```python
from build123d import *

# Parameters (mm, degrees)
SKETCH1_R           = 4
BOSS_EXTRUDE1_DEPTH = 3.175
SKETCH2_R           = 12.7
SKETCH2_R_2         = 10.287
EXTRUDE_THIN1_DEPTH = 38.1
SKETCH3_R           = 12.7
SKETCH3_R_2         = 12.5
CUT_EXTRUDE2_DEPTH  = 19.05
SKETCH4_R           = 12.5
SKETCH4_R_2         = 11.95
CUT_EXTRUDE3_DEPTH  = 1.55


with BuildPart() as part:
    # Sketch1 → Boss-Extrude1 (new body)
    with BuildSketch(Plane(origin=(0, 0, 0), x_dir=(1, 0, 0), z_dir=(0, 1, 0))):
        with BuildLine():
            Line((-8.519418994, 80.459709497), (-46.619418994, 4.259709497))
            ThreePointArc((-46.619418994, 4.259709497), (-47.625, 0), (-46.619418994, -4.259709497))
            Line((-46.619418994, -4.259709497), (-8.519418994, -80.459709497))
            ThreePointArc((-8.519418994, -80.459709497), (0, -85.725), (8.519418994, -80.459709497))
            Line((8.519418994, -80.459709497), (46.619418994, -4.259709497))
            ThreePointArc((46.619418994, -4.259709497), (47.625, 0), (46.619418994, 4.259709497))
            Line((46.619418994, 4.259709497), (8.519418994, 80.459709497))
            ThreePointArc((8.519418994, 80.459709497), (0, 85.725), (-8.519418994, 80.459709497))
        make_face()
        with Locations((0, 76.2)):
            Circle(SKETCH1_R, mode=Mode.SUBTRACT)
        with Locations((0, -76.2)):
            Circle(SKETCH1_R, mode=Mode.SUBTRACT)
        with Locations((-38.1, 0)):
            Circle(SKETCH1_R, mode=Mode.SUBTRACT)
        with Locations((38.1, 0)):
            Circle(SKETCH1_R, mode=Mode.SUBTRACT)
    extrude(amount=-BOSS_EXTRUDE1_DEPTH)

    # Sketch2 → Extrude-Thin1 (add)
    with BuildSketch(Plane(origin=(0, 0, 0), x_dir=(1, 0, 0), z_dir=(0, 1, 0))):
        Circle(SKETCH2_R)
        Circle(SKETCH2_R_2, mode=Mode.SUBTRACT)
    extrude(amount=EXTRUDE_THIN1_DEPTH)

    # Sketch3 → Cut-Extrude2 (cut)
    with BuildSketch(Plane(origin=(0, 38.1, 0), x_dir=(1, 0, 0), z_dir=(0, 1, 0))):
        Circle(SKETCH3_R)
        Circle(SKETCH3_R_2, mode=Mode.SUBTRACT)
    extrude(amount=-CUT_EXTRUDE2_DEPTH, mode=Mode.SUBTRACT)

    # Sketch4 → Cut-Extrude3 (cut)
    with BuildSketch(Plane(origin=(0, 35.063199876, 0), x_dir=(-1, 0, 0), z_dir=(0, -1, 0))):
        Circle(SKETCH4_R)
        Circle(SKETCH4_R_2, mode=Mode.SUBTRACT)
    extrude(amount=-CUT_EXTRUDE3_DEPTH, mode=Mode.SUBTRACT)


solid = part.part
```
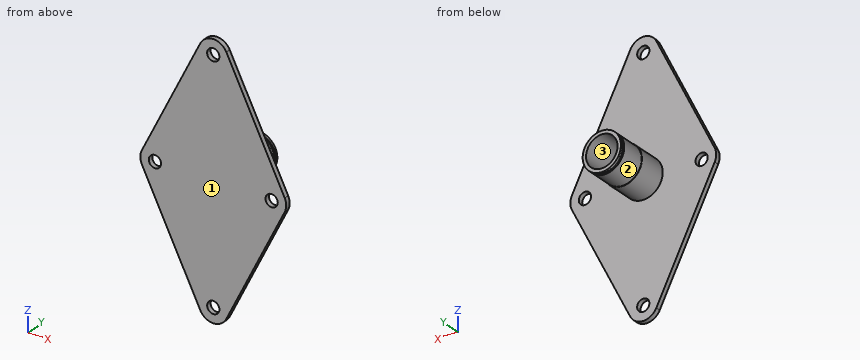
Here's how the part is built. I have some questions about the finished solid (model axes, mm). Face numbers are marked on the shaded views. Give positions to 0.01 mm unless a question says otherwise; leave off trailing zeros. Loops run counter-clockwise (first coordinate to the right, second up) from the corner with the lowest first, then second, coordinate; pieces in that order, holes last. Notation, with made-up numbers: M 37.5,25 L 54.5,25 A34 cw 54.5,60 Z; hole C 89,84.5 d3. An arc over 180 degrees is marked long. Return JSON: item names as keys, results as strings.
Item 1: Imagine slicing it at B-B on x = -38.1. List the corners of the cut face in (y, z) for me (3 decimals), then the cut area to 3 significant figures.
A:
{"outline": "M -3.175,-21.299 L 0,-21.299 L 0,-4 L -3.175,-4 Z; M -3.175,4 L 0,4 L 0,21.299 L -3.175,21.299 Z", "area": "110 mm^2"}
Item 2: Thinking about a two-plate mould opening in Z: for the marked faces 1, 2 and 3, which applies, released by +Z, released by -Z, zero draft, split by the parting line, or undercut?
A:
{"face 1": "zero draft", "face 2": "split by the parting line", "face 3": "undercut"}
Item 3: Please list where these lines run through material, in increasing order: line 1 (Z direction, x = 0, y = 30); line 2 (Y direction, x = 18, z = -46.5) (3 decimals); line 3 (X direction, y = 0.5, z = -1.5).
A:
{"line 1": "z = -12.5 to -10.29, 10.29 to 12.5", "line 2": "y = -3.175 to 0", "line 3": "x = -12.61 to -10.18, 10.18 to 12.61"}
Item 4: Imagine slicing it at C-C on z = 76.2. List the corners of the cut face in (x, y) for me (3 decimals), then the cut area to 3 significant figures.
A:
{"outline": "M -10.649,-3.175 L -4,-3.175 L -4,0 L -10.649,0 Z; M 4,-3.175 L 10.649,-3.175 L 10.649,0 L 4,0 Z", "area": "42.2 mm^2"}
Item 5: I'm going to push flat-ended pins straight in: pin 1 Ø10.5 at (x, z) = (0, 76.2) entering from +Y; pin 2 Ø2 at (y, z) = (14.5, 0) entering from +X; pin 3 Ø7 at (x, z) = (0, -76.2) entering from -Y; pin 4 Ø5 at (x, y) = (-10.5, 26) entering from -Z. Where does each tip first touch, or does it pass through?
A:
{"pin 1": "stops at y = 0", "pin 2": "stops at x = 12.7", "pin 3": "passes through", "pin 4": "stops at z = -9.6"}
Item 6: Imagine slicing it at A-A on z = 0. State how many separate pieces and enclosed holes the cut face has, then the cut area to 3 significant figures.
A:
{"separate pieces": "3", "enclosed holes": "0", "area": "426 mm^2"}
Item 7: Imagine slicing it at D-D on y = 16.5. List the corners of the cut face in (x, z) for me, then the cut area to 3 significant figures.
A:
{"outline": "C 0,0 d25.4; hole C 0,0 d20.57", "area": "174 mm^2"}
